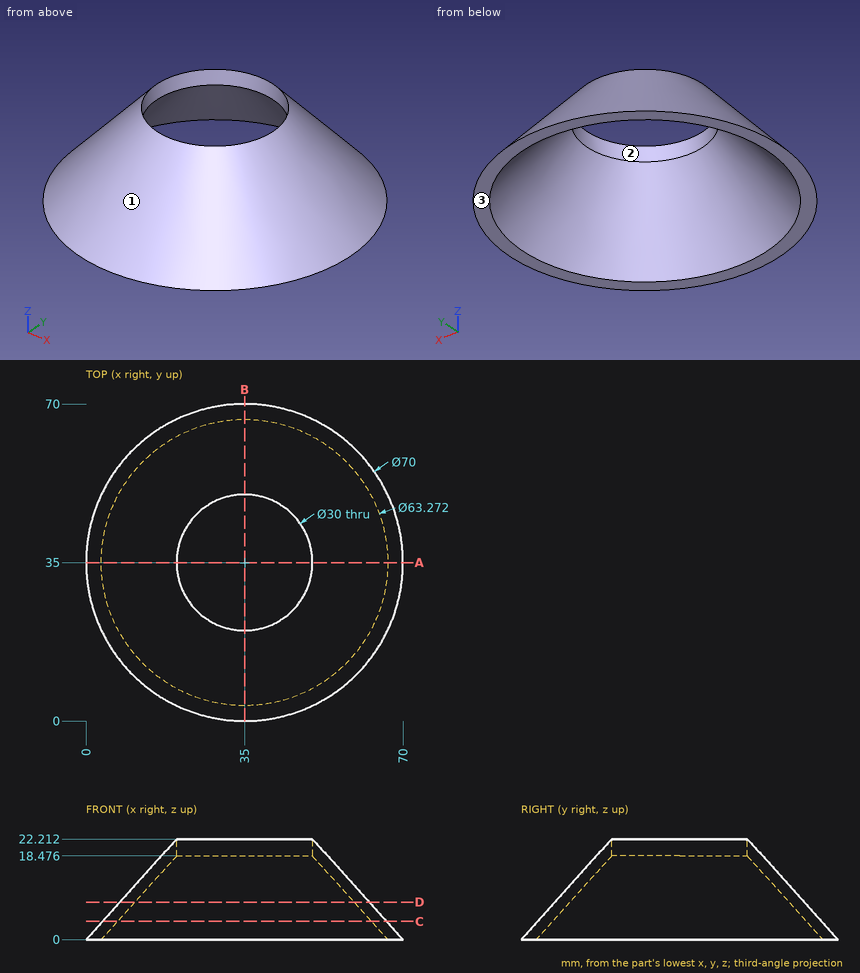
The drawing under review shows one solid part. Ordinate dimensions are in mm from its lowest x, y, z. Give positions to 0.01 mm unless a question says otherwise; leave off trailing zeros. Order: outer loops, then holes, each group sorted by start corner. A loop starts at its lowest first (then second) coordinate and runs counter-clockwise, first axis right, second up. Notation, with made-up numbers: M 29,2.25 L 41,2.25 A32 cw 41,41.25 Z; hole C -1,25.25 d4. An arc over 180 degrees is marked long. Answer in a Markdown table with one row per item. Add a question column.
1. Mouldability with a two-part tool opening along X and no side actions: class the marked faces 1, 2 and 3 as released by +X, released by -X, zero draft, split by the parting line, or undercut.
2. Add section A-A on y = 35. State the section outline as (x, z) points, plus the area to 3 significant figures.
3. Add section C-C on z = 4. State the section outline as (x, y) points.
4. Add section D-D on z = 8.25. State the section outline as (x, y) points (1 decimal), plus the area to 3 significant figures.
5. To check wall thickness, follow line 1 along X through (y, z) = (35, 21.25); line 2 along Y through (x, z) = (35, 20.9); line 3 along X through (y, z) = (37.5, 4.5). State the ranges of each line that lie inside material, in increasing order.
6. For pin 1 Ø10 at (y, z) = (46.5, 20) entering from -X; pin 2 Ø2 at (x, z) = (24.5, 10) entering from -Y; pin 3 Ø3 at (x, z) = (58, 11) entering from -Y; pin 4 Ø4 at (x, y) = (23.5, 25.5) entering from +Z, all flat-tipped, find the tip position at first contact; note any pin that passes through.
The answers:
| question | item | result |
|---|---|---|
| 1 | face 1 | split by the parting line |
| 1 | face 2 | undercut |
| 1 | face 3 | zero draft |
| 2 | outline | M 0,0 L 3.36,0 L 20,18.48 L 20,22.21 Z; M 50,18.48 L 66.64,0 L 70,0 L 50,22.21 Z |
| 2 | area | 137 mm2 |
| 3 | outline | C 35,35 d62.8; hole C 35,35 d56.07 |
| 4 | outline | C 35,35 d55.1; hole C 35,35 d48.4 |
| 4 | area | 547 mm2 |
| 5 | line 1 | 19.13 to 20, 50 to 50.87 |
| 5 | line 2 | 18.82 to 20, 50 to 51.18 |
| 5 | line 3 | 4.15 to 7.53, 62.47 to 65.85 |
| 6 | pin 1 | x = 16.13 |
| 6 | pin 2 | y = 10.15 |
| 6 | pin 3 | y = 20.95 |
| 6 | pin 4 | z = 22.21 |
